Design review of the part shown in the three views and the two pictorial views. Dimensions are in mm from the part's minimum x, y and z. Coordinates: 2 decimals unless noted, no trailing zeros. Loops run counter-clockwise (first coordinate to the right, second up) from the corner with the lowest first, then second, coordinate; pieces in that order, holes last.
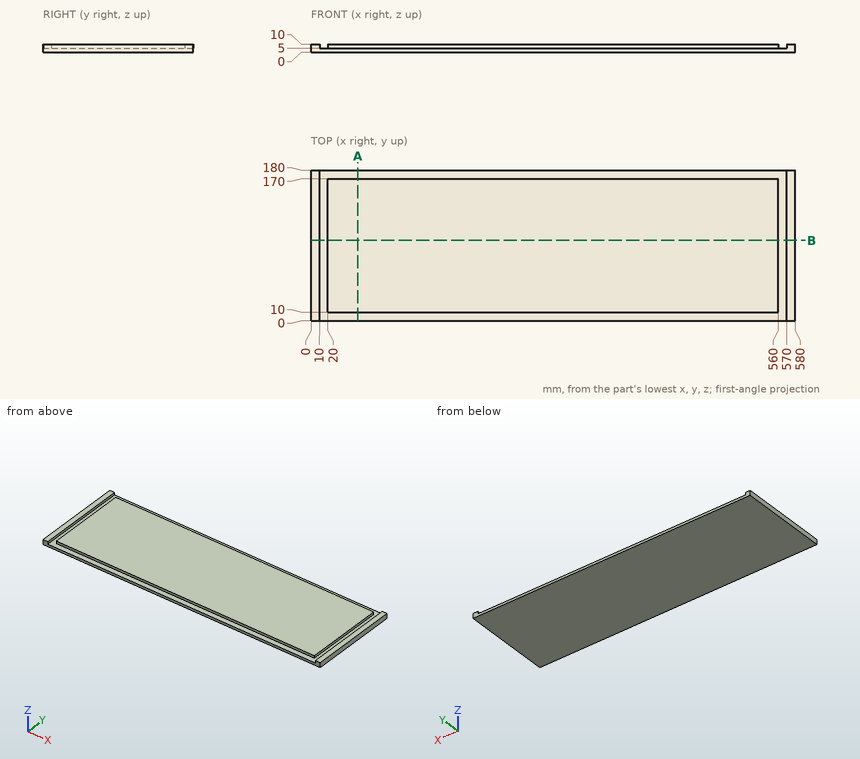
Q1. Consider section B-B (y = 96). State the section outline as (x, z) points, then the cut area to 3 significant figures.
Q2. For pin 1 Ø1.5 at (x, y) = (331, 158) entering from -Z; pin 2 Ø1.5 at (x, z) = (173, 6.5) entering from -Y, all flat-tipped, find the tip position at first contact; note any pin that passes through.
Q3. Wall thickness on probe 1 along X at (y, z) = (55, 9.25); probe 2 along Y at (x, z) = (422, 6); probe 3 along X at (y, z) = (8, 7): over which ranges is each line inside the solid? List them lowest first.
Q4. Consider section A-A (x = 56). State the section outline as (y, z) points.
Model answer:
1. outline: (0, 0) - (580, 0) - (580, 10) - (570, 10) - (570, 5) - (560, 5) - (560, 10) - (20, 10) - (20, 5) - (10, 5) - (10, 10) - (0, 10) - close
1. area: 5,700 mm2
2. pin 1: stops at z = 0
2. pin 2: stops at y = 10
3. probe 1: x = 0 to 10, 20 to 560, 570 to 580
3. probe 2: y = 10 to 170
3. probe 3: x = 0 to 10, 570 to 580
4. outline: (0, 0) - (180, 0) - (180, 5) - (170, 5) - (170, 10) - (10, 10) - (10, 5) - (0, 5) - close
